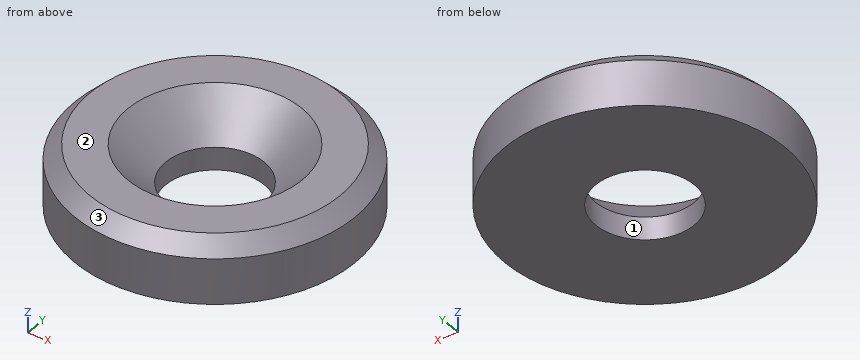
Autodesk Inventor part; units mm, degrees
ref_plane "YZ Plane" through (0, 0, 0) normal (1, 0, 0) x (0, 1, 0)
ref_plane "XZ Plane" through (0, 0, 0) normal (0, 1, 0) x (-1, 0, 0)
ref_plane "XY Plane" through (0, 0, 0) normal (0, 0, 1) x (1, 0, 0)
sketch "Sketch1" plane through (0, 0, 0) normal (0, 0, 1) x (1, 0, 0)
  circle A0 centre (0, 0) radius 9.25
  dimension "d0" = 18.5
extrude "Extrusion1" add sketch "Sketch1" along normal blind 4
sketch "Sketch2" plane through (0, 0, 4) normal (0, 0, 1) x (1, 0, 0)
  circle A0 centre (0, 0) radius 9.25
hole "Hole1" at (0, 0, 4) direction (0, 0, -1) diameter 6.5 depth 4 tip angle 118 countersink diameter 11.5 countersink angle 90
chamfer "Chamfer1" distance 1 angle 45 1 edges at (-9.25, 0, 4)
properties part number "ARRUELA ESPECIAL DAS RODAS(31)" material "Carbon Steel"
Check sheet for the modelled part. Datum: model origin and axes. Units: mm. Face numbers are marked on the shaded views. Coordinates: 2 decimals unless noted, no trailing zeros. Order: outer loops, then holes, each group sorted by start corner. A loop starts at its lowest first (then second) coordinate and runs counter-clockwise, first axis right, second up. Notation, with made-up numbers: (21, 36.5) -> (62, 36.5) arc R21 ccw to (62, 59.5) -> close; hole circle Ø4 at (-9.5, 62.25). An arc over 180 degrees is marked (long way). Write item = value, one per line. Start each with the question number.
1) Go/stop test with flat-tipped pins: P1, Ø7.5, axis at x = 0, y = 0, coming from the -Z side; P2, Ø1.5, axis at x = -4.5, y = 1, coming from the +Z side; P3, Ø5, axis at x = -2, y = -2.5, coming from the +Z side; P4, Ø1, axis at x = 5, z = 2, coming from the -Y side. Record where each tip stops, or that it passes through.
2) Mould release check, pull along Y, two halves, no side actions. Record for the marked faces 1, 2 and 3: +Y half, -Y half, draft (parallel to the pull), parting line (faces both ways), or undercut.
3) Material ranges on L1, parallel to Y at x = 0, z = 0.5; L2, parallel to Y at x = 3.25, z = 3.35; L3, parallel to X at y = -7.25, z = 1.1, recorded low to high.
4) Cross-section at D-D (z = 0.6). Enter the section's corners in (x, y), then the cut area to 3 significant figures.
5) Cross-section at C-C (z = 2). Enter the section's corners in (x, y).
6) Cross-section at A-A (x = 0). Enter the section's corners in (y, z).
Ans:
q1.P1 = 0
q1.P2 = 3.61
q1.P3 = 3.95
q1.P4 = -8.08
q2.face_1 = undercut
q2.face_2 = draft
q2.face_3 = parting line
q3.L1 = -9.25 to -3.25, 3.25 to 9.25
q3.L2 = -8.29 to -3.93, 3.93 to 8.29
q3.L3 = -5.74 to 5.74
q4.outline = circle Ø18.5 at (0, 0); hole circle Ø6.5 at (0, 0)
q4.area = 236 mm²
q5.outline = circle Ø18.5 at (0, 0); hole circle Ø7.5 at (0, 0)
q6.outline = (-9.25, 0) -> (-3.25, 0) -> (-3.25, 1.5) -> (-5.75, 4) -> (-8.25, 4) -> (-9.25, 3) -> close; (3.25, 0) -> (9.25, 0) -> (9.25, 3) -> (8.25, 4) -> (5.75, 4) -> (3.25, 1.5) -> close
